Input: part model. Units: mm. Frame: model coordinates. A direction names the side the tool comes from. Give positions to 0.01 mm unless a question says otherwise; leave off trailing zeros. Loops run counter-clockwise (first coordinate to the right, second up) from the corner with the lowest first, then second, coordinate; pieces in that order, holes last. Notation, with made-up numbers: (-4.5, -4.5) -> (32.5, -4.5) arc R10 cw to (32.5, 1.5) -> close; hole circle Ø3 at (-17.75, 54). An arc over 180 degrees is marked (long way). Answer as a JSON object with one key per item and string values.
```python
from build123d import *

# Parameters (mm, degrees)
SKETCH_2_R          = 6.05
SKETCH_2_R_2        = 2.05
EXTRUDE_1_DEPTH     = 5
EXTRUDE_1_2_DEPTH   = 5
EXTRUDE_1_3_DEPTH   = 5
EXTRUDE_1_4_DEPTH   = 5
SKETCH_6_R          = 2.05
EXTRUDE_1_5_DEPTH   = 5
SKETCH_8_W          = 18.5
SKETCH_8_H          = 16
SKETCH_8_W_2        = 10.5
SKETCH_8_H_2        = 5.2
SKETCH_8_W_3        = 14
SKETCH_8_H_3        = 9
CUT_EXTRUDE_2_DEPTH = 153.920706577


with BuildPart() as part:
    # 草图2 → Extrude 1 (new body)
    with BuildSketch(Plane(origin=(0, 0, 0), x_dir=(-1, 0, 0), z_dir=(0, -1, 0))):
        with Locations((-103.2, -9.35)):
            Circle(SKETCH_2_R)
        with Locations((-103.2, -9.35)):
            Circle(SKETCH_2_R_2, mode=Mode.SUBTRACT)
    extrude(amount=EXTRUDE_1_DEPTH)



with BuildPart() as body_2:
    # 草图2 → Extrude 1 2 (new body)
    with BuildSketch(Plane(origin=(0, 0, 0), x_dir=(-1, 0, 0), z_dir=(0, -1, 0))):
        with Locations((-63.2, -9.35)):
            Circle(SKETCH_2_R)
        with Locations((-63.2, -9.35)):
            Circle(SKETCH_2_R_2, mode=Mode.SUBTRACT)
    extrude(amount=EXTRUDE_1_2_DEPTH)


with BuildPart() as body_3:
    # 草图2 → Extrude 1 3 (new body)
    with BuildSketch(Plane(origin=(0, 0, 0), x_dir=(-1, 0, 0), z_dir=(0, -1, 0))):
        with Locations((-63.2, -64.25)):
            Circle(SKETCH_2_R)
        with Locations((-63.2, -64.25)):
            Circle(SKETCH_2_R_2, mode=Mode.SUBTRACT)
    extrude(amount=EXTRUDE_1_3_DEPTH)


with BuildPart() as body_4:
    # 草图2 → Extrude 1 4 (new body)
    with BuildSketch(Plane(origin=(0, 0, 0), x_dir=(-1, 0, 0), z_dir=(0, -1, 0))):
        with Locations((-103.2, -64.25)):
            Circle(SKETCH_2_R)
        with Locations((-103.2, -64.25)):
            Circle(SKETCH_2_R_2, mode=Mode.SUBTRACT)
    extrude(amount=EXTRUDE_1_4_DEPTH)


with BuildPart() as part_1:
    add(part.part)

    add(body_2.part)  # Extrude 1 5 merges body 2

    add(body_3.part)  # Extrude 1 5 merges body 3

    add(body_4.part)  # Extrude 1 5 merges body 4
    # 草图6 → Extrude 1 5 (add)
    with BuildSketch(Plane(origin=(0, 0, 0), x_dir=(1, 0, 0), z_dir=(0, 1, 0))):
        with BuildLine():
            Line((127.2, 1.45), (109.046152581, 1.45))
            ThreePointArc((109.046152581, 1.45), (105.271235363, 0.113689527), (103.177805284, -3.3))
            Line((103.177805284, -3.3), (63.2, -3.3))
            Line((63.2, -3.3), (49.25, -3.3))
            ThreePointArc((49.25, -3.3), (44.972003974, -5.072003974), (43.2, -9.35))
            Line((43.2, -9.35), (43.2, -64.3))
            ThreePointArc((43.2, -64.3), (44.957359313, -68.542640687), (49.2, -70.3))
            Line((49.2, -70.3), (103.2, -70.3))
            ThreePointArc((103.2, -70.3), (105.311182702, -73.645742753), (109.046152581, -74.95))
            Line((109.046152581, -74.95), (127.2, -74.95))
            ThreePointArc((127.2, -74.95), (131.442640687, -73.192640687), (133.2, -68.95))
            Line((133.2, -68.95), (133.2, -4.55))
            ThreePointArc((133.2, -4.55), (131.442640687, -0.307359313), (127.2, 1.45))
        make_face()
        with Locations(Location((103.2, -9.35, 0), (0, 0, 270))):
            Circle(SKETCH_6_R, mode=Mode.SUBTRACT)
        with Locations(Location((103.2, -64.25, 0), (0, 0, 270))):
            Circle(SKETCH_6_R, mode=Mode.SUBTRACT)
        with Locations(Location((63.2, -64.25, 0), (0, 0, 270))):
            Circle(SKETCH_6_R, mode=Mode.SUBTRACT)
        with Locations(Location((63.2, -9.35, 0), (0, 0, 90))):
            Circle(SKETCH_6_R, mode=Mode.SUBTRACT)
    extrude(amount=-EXTRUDE_1_5_DEPTH)

    # 草图8 → 切除-拉伸2 (cut, through all)
    with BuildSketch(Plane.XZ):
        with BuildLine():
            Line((67.2, 13.45), (67.2, 40.45))
            Line((67.2, 40.45), (60.461737691, 40.45))
            ThreePointArc((60.461737691, 40.45), (57.9, 45.7), (55.338262309, 40.45))
            Line((55.338262309, 40.45), (49.2, 40.45))
            Line((49.2, 40.45), (49.2, 13.45))
            Line((49.2, 13.45), (51.063508327, 13.45))
            ThreePointArc((51.063508327, 13.45), (53, 5.95), (54.936491673, 13.45))
            Line((54.936491673, 13.45), (67.2, 13.45))
        make_face()
        with Locations((117.45, 10.45)):
            Rectangle(SKETCH_8_W, SKETCH_8_H)
        with BuildLine():
            Line((108.2, 20.95), (125.2, 20.95))
            Line((125.2, 20.95), (125.2, 25.8))
            ThreePointArc((125.2, 25.8), (129.203625856, 29.497066152), (124.2, 31.656011826))
            Line((124.2, 31.656011826), (124.2, 35.143988174))
            ThreePointArc((124.2, 35.143988174), (129.25, 37.85), (124.2, 40.556011826))
            Line((124.2, 40.556011826), (124.2, 44.043988174))
            ThreePointArc((124.2, 44.043988174), (129.25, 46.75), (124.2, 49.456011826))
            Line((124.2, 49.456011826), (124.2, 52.943988174))
            ThreePointArc((124.2, 52.943988174), (129.25, 55.65), (124.2, 58.356011826))
            Line((124.2, 58.356011826), (124.2, 63.75))
            Line((124.2, 63.75), (122.2, 63.75))
            Line((122.2, 63.75), (111.7, 63.75))
            Line((111.7, 63.75), (109.7, 63.75))
            Line((109.7, 63.75), (109.7, 30.95))
            Line((109.7, 30.95), (108.2, 30.95))
            Line((108.2, 30.95), (108.2, 20.95))
        make_face()
        with Locations((116.95, 67.35)):
            Rectangle(SKETCH_8_W_2, SKETCH_8_H_2)
        with Locations((82.2, 68.85)):
            Rectangle(SKETCH_8_W_3, SKETCH_8_H_3)
    extrude(amount=CUT_EXTRUDE_2_DEPTH, mode=Mode.SUBTRACT)


solid = part_1.part
```
Q1. Ray query, line 1 along Z through (x, y) = (126, -3.35); line 2 along Z through (x, y) = (112, -2.05); line 3 along X through (y, z) = (-1.75, 25). Return the intervals inside material, ascending.
Evaluation:
{"line 1": "z = -1.45 to 2.45, 18.45 to 25.7, 32.2 to 34.6, 41.1 to 43.5, 50 to 52.4, 58.9 to 74.95", "line 2": "z = -1.45 to 2.45, 18.45 to 20.95, 63.75 to 64.75, 69.95 to 74.95", "line 3": "x = 43.2 to 49.2, 67.2 to 108.2, 125.2 to 133.2"}
Q2. Section C-C, the plane x = 63.2. Return the cut outline in (y, z).
Evaluation:
{"outline": "(-5, 3.3) -> (0, 3.3) -> (0, 7.3) -> (-5, 7.3) -> close; (-5, 11.4) -> (0, 11.4) -> (0, 13.45) -> (-5, 13.45) -> close; (-5, 40.45) -> (0, 40.45) -> (0, 62.2) -> (-5, 62.2) -> close; (-5, 66.3) -> (0, 66.3) -> (0, 70.3) -> (-5, 70.3) -> close"}
Q3. Access query for faces 4 (the flat face through (82, -2, 64.35)), 5 (the cylindrical face through (105.316, -2.465, -0.149)), 6 (the flat face through (96, -2, 70.3)), 7 (the flat face through (118, -2, 74.95)), 8 (the flat face through (61, -2, 13.45)). Directions: +Z, -Z, +X, -X, +Y, -Y. A direction counts if a zero-diameter tool reaches every point of the face in a straight line with its end or side. Return the directions, or none.
Evaluation:
{"face 4": "+Z, +Y, -Y", "face 5": "-Z, -X, +Y, -Y", "face 6": "+Z, -X, +Y, -Y", "face 7": "+Z, +X, -X, +Y, -Y", "face 8": "+Y, -Y"}
Q4. Section D-D, the plane z = 42.45. Return the cut outline in (x, y), then the cut area to 3 significant figures.
Evaluation:
{"outline": "(43.2, -5) -> (54.65, -5) -> (54.65, 0) -> (43.2, 0) -> close; (61.15, -5) -> (109.7, -5) -> (109.7, 0) -> (61.15, 0) -> close; (124.2, -5) -> (133.2, -5) -> (133.2, 0) -> (124.2, 0) -> close", "area": "345 mm2"}
Q5. Pin query (flat end, axial travel): pin 1 (1.5 mm diameter, centred on y = -3.5, z = 68.5, fed in from -X); pin 2 (1.5 mm diameter, centred on x = 84.5, y = -2, fed in from +Z); pin 3 (2.5 mm diameter, centred on x = 51, y = -2, fed in from -Z). Return the tip coordinate at first contact, or that it passes through.
Evaluation:
{"pin 1": "stops at x = 44.29", "pin 2": "stops at z = 64.35", "pin 3": "stops at z = 3.3"}
Q6. Draft query along Z for faces 1 (the cylindrical face through (44.911, -2.465, 68.496)), 2 (the flat face through (133.2, -2, 37)), 3 (the cylindrical face through (58, -2.5, 45.7)). Return one class per face: +Z half, -Z half, draft (parallel to the pull), parting line (faces both ways), or undercut.
Evaluation:
{"face 1": "+Z half", "face 2": "draft", "face 3": "undercut"}
Q7. Section B-B, the plane z = 28.95. Return the cut outline in (x, y).
Evaluation:
{"outline": "(43.2, -5) -> (49.2, -5) -> (49.2, 0) -> (43.2, 0) -> close; (67.2, -5) -> (108.2, -5) -> (108.2, 0) -> (67.2, 0) -> close; (129.25, -5) -> (133.2, -5) -> (133.2, 0) -> (129.25, 0) -> close"}
Q8. Section A-A, the plane z = 61. Return the cut outline in (x, y).
Evaluation:
{"outline": "(43.2, -5) -> (109.7, -5) -> (109.7, 0) -> (43.2, 0) -> close; (124.2, -5) -> (133.2, -5) -> (133.2, 0) -> (124.2, 0) -> close"}
